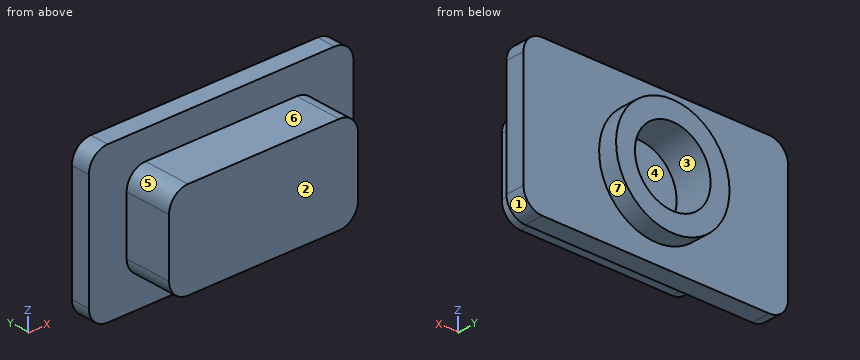
from build123d import *

# Parameters (mm, degrees)
SALIENTE_EXTRUIR1_DEPTH = 2.5
SALIENTE_EXTRUIR2_DEPTH = 1
CROQUIS3_R              = 3
SALIENTE_EXTRUIR3_DEPTH = 1
CROQUIS4_R              = 2
CORTAR_EXTRUIR1_DEPTH   = 2


with BuildPart() as part:
    # Croquis1 → Saliente-Extruir1 (new body)
    with BuildSketch(Plane(origin=(0, 0, 0), x_dir=(1, 0, 0), z_dir=(0, 1, 0))):
        with BuildLine():
            Line((-4, -2.5), (4, -2.5))
            ThreePointArc((4, -2.5), (4.707106781, -2.207106781), (5, -1.5))
            Line((5, -1.5), (5, 1.5))
            ThreePointArc((5, 1.5), (4.707106781, 2.207106781), (4, 2.5))
            Line((4, 2.5), (-4, 2.5))
            ThreePointArc((-4, 2.5), (-4.707106781, 2.207106781), (-5, 1.5))
            Line((-5, 1.5), (-5, -1.5))
            ThreePointArc((-5, -1.5), (-4.707106781, -2.207106781), (-4, -2.5))
        make_face()
    extrude(amount=SALIENTE_EXTRUIR1_DEPTH)

    # Croquis2 → Saliente-Extruir2 (add)
    with BuildSketch(Plane(origin=(0, 2.5, 0), x_dir=(1, 0, 0), z_dir=(0, 1, 0))):
        with BuildLine():
            Line((-6, -4), (6, -4))
            ThreePointArc((6, -4), (6.707106781, -3.707106781), (7, -3))
            Line((7, -3), (7, 3))
            ThreePointArc((7, 3), (6.707106781, 3.707106781), (6, 4))
            Line((6, 4), (-6, 4))
            ThreePointArc((-6, 4), (-6.707106781, 3.707106781), (-7, 3))
            Line((-7, 3), (-7, -3))
            ThreePointArc((-7, -3), (-6.707106781, -3.707106781), (-6, -4))
        make_face()
    extrude(amount=SALIENTE_EXTRUIR2_DEPTH)

    # Croquis3 → Saliente-Extruir3 (add)
    with BuildSketch(Plane(origin=(0, 3.5, 0), x_dir=(1, 0, 0), z_dir=(0, 1, 0))):
        with Locations(Location((0, 0, 0), (0, 0, 270))):
            Circle(CROQUIS3_R)
    extrude(amount=SALIENTE_EXTRUIR3_DEPTH)

    # Croquis4 → Cortar-Extruir1 (cut)
    with BuildSketch(Plane(origin=(0, 4.5, 0), x_dir=(1, 0, 0), z_dir=(0, 1, 0))):
        with Locations(Location((0, 0, 0), (0, 0, 270))):
            Circle(CROQUIS4_R)
    extrude(amount=-CORTAR_EXTRUIR1_DEPTH, mode=Mode.SUBTRACT)


solid = part.part
Model file for the job. Use its own axes, mm. Face numbers are marked on the shaded views. A direction names the side the tool comes from. Round coordinates to 2 decimals unless told otherwise and drop trailing zeros. Loops run counter-clockwise (first coordinate to the right, second up) from the corner with the lowest first, then second, coordinate; pieces in that order, holes last.
1. Band-saw the part on D-D, the plane x = 0. List the corners of the cut face in (y, z), and give its area (3 significant figures).
Check values:
outline: (0, -2.5) - (2.5, -2.5) - (2.5, -4) - (3.5, -4) - (3.5, -3) - (4.5, -3) - (4.5, -2) - (2.5, -2) - (2.5, 2) - (4.5, 2) - (4.5, 3) - (3.5, 3) - (3.5, 4) - (2.5, 4) - (2.5, 2.5) - (0, 2.5) - close
area: 18.5 mm2
2. Tool access for the marked faces 5, 6 and 7: list every direction of +Z, -Z, +X, -X, +Y, -Y with a clear straight run to the whole face (end or side of a thin tool).
Check values:
face 5: +Z, -X, -Y
face 6: +Z, +X, -X, -Y
face 7: +Y
3. Band-saw the part on B-B, the plane z = 0. List the corners of the cut face in (x, y), and give its area (3 significant figures).
Check values:
outline: (-7, 2.5) - (-5, 2.5) - (-5, 0) - (5, 0) - (5, 2.5) - (7, 2.5) - (7, 3.5) - (3, 3.5) - (3, 4.5) - (2, 4.5) - (2, 2.5) - (-2, 2.5) - (-2, 4.5) - (-3, 4.5) - (-3, 3.5) - (-7, 3.5) - close
area: 37.0 mm2
4. Drop flat-ended pins along their axis: P1, Ø1.5, axis at x = 1, z = 0, coming from the +Y side; P2, Ø1.5, axis at y = 1.5, z = 2, coming from the -X side; P3, Ø1.2, axis at x = 0.5, y = 0.5, coming from the -Z side; P4, Ø3, axis at x = 5, z = 0, coming from the -Y side. Give the stop position or say it passes through.
Check values:
P1: stops at y = 2.5
P2: stops at x = -5
P3: stops at z = -2.5
P4: stops at y = 0
5. Wall check: probe 1 along X at (y, z) = (3.7, 0); probe 2 along X at (y, z) = (3.4, 0); probe 3 along Y at (x, z) = (-3.25, 0.75). Give the ranges that are in metal, low to high.
Check values:
probe 1: x = -3 to -2, 2 to 3
probe 2: x = -7 to -2, 2 to 7
probe 3: y = 0 to 3.5
6. Band-saw the part on A-A, the plane y = 1.1. List the corners of the cut face in (x, z).
Check values:
outline: (-5, -1.5) arc R1 ccw to (-4, -2.5) - (4, -2.5) arc R1 ccw to (5, -1.5) - (5, 1.5) arc R1 ccw to (4, 2.5) - (-4, 2.5) arc R1 ccw to (-5, 1.5) - close
7. Mould opens along X. For the marked faces 1, 2, 3 and 4 say: +X half, -X half, draft (parallel to the pull), parting line (faces both ways), or undercut.
Check values:
face 1: +X half
face 2: draft
face 3: undercut
face 4: undercut
8. Band-saw the part on C-C, the plane y = 2.85. List the corners of the cut face in (x, z), and give its area (3 significant figures).
Check values:
outline: (-7, -3) arc R1 ccw to (-6, -4) - (6, -4) arc R1 ccw to (7, -3) - (7, 3) arc R1 ccw to (6, 4) - (-6, 4) arc R1 ccw to (-7, 3) - close; hole circle Ø4 at (0, 0)
area: 98.6 mm2
